Autodesk Inventor part; units mm, degrees
ref_plane "YZ Plane" through (0, 0, 0) normal (1, 0, 0) x (0, 1, 0)
ref_plane "XZ Plane" through (0, 0, 0) normal (0, 1, 0) x (-1, 0, 0)
ref_plane "XY Plane" through (0, 0, 0) normal (0, 0, 1) x (1, 0, 0)
sketch "Sketch1" plane through (0, 0, 0) normal (1, 0, 0) x (0, 1, 0)
  line L0 (-25, 75) -> (-25, -75)
  line L1 (-25, -75) -> (12.3, -75)
  line L2 (25, -50) -> (25, 50)
  line L3 (12.3, 75) -> (-25, 75)
  line L4 (12.3, 75) -> (12.3, 50)
  line L5 (12.3, 50) -> (25, 50)
  line L6 (12.3, -75) -> (12.3, -50)
  line L7 (12.3, -50) -> (25, -50)
  circle A0 centre (-15, 50) radius 2.95
  circle A1 centre (-15, -50) radius 2.95
  point P0 (0, 0)
  point P1 (25, 0)
  point P2 (0, 75)
  point P3 (18.65, 50)
  point P4 (18.65, -50)
  point P5 (25, 0)
  dimension "d0" = 150
  dimension "d2" = 12.7
  dimension "d3" = 25
  dimension "d4" = 12.7
  dimension "d5" = 25
  dimension "d6" = 50
  dimension "d7" = 5.9
  dimension "d8" = 5.9
  dimension "d9" = 10
extrude "Extrusion1" add sketch "Sketch1" along normal blind 6.35
properties part number "SideV1"
Work out the finished part from the listing and answer in its coordinate system (mm). A direction names the side the tool comes from. Round coordinates to 2 decimals unless told otherwise and drop trailing zeros. Write each loop counter-clockwise with the first axis right and the second up, starting at its lowest first coordinate (ties: lowest second). Pieces come first, ordered by that corner, then holes.
1) A tool of negligible diameter and unlimited length cuts with its end or side. For faces 4 (the flat face through (3, 12.3, -63)), 5 (the flat face through (3, -7, -75)), 6 (the flat face through (3, 19, 50)), from which of +Z, -Z, +X, -X, +Y, -Y can it reach the whole face along a straight path? Write none if from no direction.
2) The mould has two halves that part along Z. Classify faces 1 (the cylindrical face through (3.13, -15.64, -47.12)), 2 (the flat face through (3, 19, -50)), 3 (the flat face through (6.35, 0, 1)): pulls with the +Z half, pulls with the -Z half, needs draft (parallel to the pull), parting line crosses it, or undercut.
3) A cutting plane is placed at A-A (x = 4.75). Give the vertices of the cut face in (y, z), plus the area to 3 significant figures.
4) A cutting plane is placed at B-B (y = -15). Give the vertices of the cut face in (x, z), plus the area to 3 significant figures.
5) Given pin 1 Ø1 at (y, z) = (-15.5, -17) entering from -X; pin 2 Ø3 at (x, y) = (4.5, 19) entering from -Z; pin 3 Ø3 at (x, y) = (2, 18.5) entering from +Z, each flat-ended and moving along its own axis, determine where each tip first touches the part or whether it passes through.
6) Straight lines are drawn through the part: line 1 (Z direction, x = 4, y = -15); line 2 (Z direction, x = 1.75, y = -14); line 3 (Y direction, x = 5.5, z = 53). For each, find the intervals that lie inside material, in ascending order.
7) A cutting plane is placed at C-C (z = -66). Give the vertices of the cut face in (x, y), plus the area to 3 significant figures.
Completed:
1. face 4: -Z, +X, -X, +Y
1. face 5: -Z, +X, -X, +Y, -Y
1. face 6: +Z, +X, -X, +Y
2. face 1: undercut
2. face 2: pulls with the -Z half
2. face 3: needs draft
3. outline: (-25, -75) - (12.3, -75) - (12.3, -50) - (25, -50) - (25, 50) - (12.3, 50) - (12.3, 75) - (-25, 75) - close; hole circle Ø5.9 at (-15, -50); hole circle Ø5.9 at (-15, 50)
3. area: 6,810 mm2
4. outline: (0, -75) - (6.35, -75) - (6.35, -52.95) - (0, -52.95) - close; (0, -47.05) - (6.35, -47.05) - (6.35, 47.05) - (0, 47.05) - close; (0, 52.95) - (6.35, 52.95) - (6.35, 75) - (0, 75) - close
4. area: 878 mm2
5. pin 1: stops at x = 0
5. pin 2: stops at z = -50
5. pin 3: stops at z = 50
6. line 1: z = -75 to -52.95, -47.05 to 47.05, 52.95 to 75
6. line 2: z = -75 to -52.78, -47.22 to 47.22, 52.78 to 75
6. line 3: y = -25 to 12.3
7. outline: (0, -25) - (6.35, -25) - (6.35, 12.3) - (0, 12.3) - close
7. area: 237 mm2
